Could you check a few things on this model? Use its own coordinates, in mm. A direction names the side the tool comes from. Coordinates: 2 decimals unless noted, no trailing zeros. Loops run counter-clockwise (first coordinate to the right, second up) from the corner with the lowest first, then second, coordinate; pieces in that order, holes last. Notation, with made-up numbers: (-19.75, 59.25) -> (20.25, 59.25) arc R25 ccw to (20.25, 71.25) -> close; hole circle Ø9 at (-2, 68). An arc over 180 degrees is marked (long way). One line per question, with ' | ' between items.
from build123d import *

# Parameters (mm, degrees)
BOSS_EXTRUDE1_DEPTH     = 64
SKETCH2_W               = 50
SKETCH2_H               = 7.2
CUT_EXTRUDE1_DEPTH      = 12.5
CUT_EXTRUDE1_DEPTH_BACK = 4.5
SKETCH3_W               = 16
SKETCH3_H               = 8
CUT_EXTRUDE2_DEPTH      = 64


with BuildPart() as part:
    # Sketch1 → Boss-Extrude1 (new body)
    with BuildSketch(Plane(origin=(0, 0, 0), x_dir=(0, 0, -1), z_dir=(1, 0, 0))):
        Polygon((0.359176952, -3.317134482), (0.359176952, 0.182865518), (12.359176952, 0.182865518), (17.818730466, -14.817134482), (12.359176952, -14.817134482), (0.359176952, -14.817134482), (0.359176952, -11.317134482), (7.559176952, -11.317134482), (7.559176952, -3.317134482), align=None)
    extrude(amount=BOSS_EXTRUDE1_DEPTH)

    # Sketch2 → Cut-Extrude1 (cut, two sides)
    with BuildSketch(Plane(origin=(0, -11.317134482, 0), x_dir=(1, 0, 0), z_dir=(0, 1, 0))) as cut_extrude1_sk:
        with Locations((32, 3.959176952)):
            Rectangle(SKETCH2_W, SKETCH2_H)
    extrude(amount=CUT_EXTRUDE1_DEPTH, mode=Mode.SUBTRACT)
    extrude(cut_extrude1_sk.sketch, amount=-CUT_EXTRUDE1_DEPTH_BACK, mode=Mode.SUBTRACT)

    # Sketch3 → Cut-Extrude2 (cut)
    with BuildSketch(Plane.XY.offset(-7.559176952)):
        with Locations((33.5, -10.817134482)):
            Rectangle(SKETCH3_W, SKETCH3_H)
    extrude(amount=-CUT_EXTRUDE2_DEPTH, mode=Mode.SUBTRACT)


solid = part.part
1) If we section it at A-A on z = -4.25: Please give me the cut outline in (x, y).
Data:
outline: (0, -14.82) -> (7, -14.82) -> (7, -11.32) -> (0, -11.32) -> close; (0, -3.32) -> (7, -3.32) -> (7, 0.18) -> (0, 0.18) -> close; (57, -14.82) -> (64, -14.82) -> (64, -11.32) -> (57, -11.32) -> close; (57, -3.32) -> (64, -3.32) -> (64, 0.18) -> (57, 0.18) -> close
2) I'm going to push flat-ended pins straight in: pin 1 Ø2 at (x, z) = (32, -10.5) entering from -Y; pin 2 Ø5 at (y, z) = (-12.5, -7.5) entering from -X; pin 3 Ø6 at (x, z) = (11.5, -3.5) entering from +Y. Where does each tip first touch, or does it pass through?
Data:
pin 1: y = -6.82 | pin 2: x = 0 | pin 3: through
3) If we section it at C-C on x = 5: Please give me the cut outline in (y, z), and give its area (3 significant figures).
Data:
outline: (-14.82, -17.82) -> (0.18, -12.36) -> (0.18, -0.36) -> (-3.32, -0.36) -> (-3.32, -7.56) -> (-11.32, -7.56) -> (-11.32, -0.36) -> (-14.82, -0.36) -> close | area: 163 mm²
4) On a 3-axis mill with a long thin cutter (end or side, diameter ignored), from which of +Z, -Z, +X, -X, +Y, -Y can I reach the whole of each face in a straight line? I mean faces 1 (the face through (60, -2, -0.359)), 2 (the face through (57, -13, -4)), 3 (the face through (25.5, -11, -11)), 4 (the face through (3, -11.317, -4)). Say none if no direction works.
Data:
face 1: +Z, +X, -X, +Y, -Y | face 2: +Z, +Y, -Y | face 3: +Z, -Z, -Y | face 4: +Z, +X, -X
5) If we section it at B-B on y = -9.75: Please give me the cut outline in (x, z), and give its area (3 significant figures).
Data:
outline: (0, -15.97) -> (25.5, -15.97) -> (25.5, -7.56) -> (0, -7.56) -> close; (41.5, -15.97) -> (64, -15.97) -> (64, -7.56) -> (41.5, -7.56) -> close | area: 404 mm²
6) If we section it at D-D on z = -11.75: Please give me the cut outline in (x, y).
Data:
outline: (0, -14.82) -> (25.5, -14.82) -> (25.5, -6.82) -> (41.5, -6.82) -> (41.5, -14.82) -> (64, -14.82) -> (64, 0.18) -> (0, 0.18) -> close
7) I need wall thicknesses on line 1 along X through (y, z) = (-2.75, -4); line 2 along X through (y, z) = (-12.5, -10.25); line 3 along Y through (x, z) = (34, -9.5). Which ranges of each line are inside material? Lowest first, please. Write a range as from..to.
Data:
line 1: 0..7, 57..64 | line 2: 0..25.5, 41.5..64 | line 3: -6.82..0.18
8) We'd pull the mould along Y, two halves only. Please class faces 5 (the face through (33, -6.817, -11)), 6 (the face through (60, -11.317, -4)), 7 (the face through (57, -2, -4)), 8 (the face through (31.552, -5.545, -14.444)): pulls with the +Y half, pulls with the -Y half, needs draft (parallel to the pull), parting line crosses it, or undercut.
Data:
face 5: pulls with the -Y half | face 6: undercut | face 7: needs draft | face 8: pulls with the +Y half
